```python
from build123d import *

# Parameters (mm, degrees)
ESQUISSE1_W        = 20
ESQUISSE1_H        = 7
BOSS_EXTRU_1_DEPTH = 23
ESQUISSE2_W        = 5
ESQUISSE2_H        = 2.5
BOSS_EXTRU_2_DEPTH = 2.5
ESQUISSE3_W        = 3
ESQUISSE3_H        = 3
ESQUISSE3_W_2      = 20
ESQUISSE3_H_2      = 7
BOSS_EXTRU_3_DEPTH = 2
CONG_1_R           = 2


with BuildPart() as part:
    # Esquisse1 → Boss.-Extru.1 (new body)
    with BuildSketch(Plane.XY):
        with Locations((10, 3.5)):
            Rectangle(ESQUISSE1_W, ESQUISSE1_H)
    extrude(amount=BOSS_EXTRU_1_DEPTH)

    # Esquisse2 → Boss.-Extru.2 (add)
    with BuildSketch(Plane.XY.offset(23)):
        with Locations((6.25, 3.5)):
            Rectangle(ESQUISSE2_W, ESQUISSE2_H)
        with Locations((13.75, 3.5)):
            Rectangle(ESQUISSE2_W, ESQUISSE2_H)
    extrude(amount=BOSS_EXTRU_2_DEPTH)

    # Esquisse3 → Boss.-Extru.3 (add)
    # profile 1 of 3: a face of its own
    with BuildSketch(Plane(origin=(0, 0, 0), x_dir=(-1, 0, 0), z_dir=(0, 0, -1))):
        with Locations((-21.5, 8.5)):
            Rectangle(ESQUISSE3_W, ESQUISSE3_H)
    # profile 2 of 3: a face of its own
    with BuildSketch(Plane(origin=(0, 0, 0), x_dir=(-1, 0, 0), z_dir=(0, 0, -1))):
        Polygon((-20, 10), (-20, 7), (-23, 7), (-23, -3), (3, -3), (3, 10), align=None)
        with Locations((-10, 3.5)):
            Rectangle(ESQUISSE3_W_2, ESQUISSE3_H_2, mode=Mode.SUBTRACT)
    # profile 3 of 3: a face of its own
    with BuildSketch(Plane(origin=(0, 0, 0), x_dir=(-1, 0, 0), z_dir=(0, 0, -1))):
        with Locations((-10, 3.5)):
            Rectangle(ESQUISSE3_W_2, ESQUISSE3_H_2)
    extrude(amount=BOSS_EXTRU_3_DEPTH)

    # Congé1
    cong_1_edges = [part.edges().sort_by_distance(p)[0] for p in [
        (10, 7, 0),
        (20, 3.5, 0),
        (10, 0, 0),
        (0, 3.5, 0),
    ]]
    fillet(cong_1_edges, radius=CONG_1_R)


solid = part.part
```
The model under review builds one solid part; all positions refer to its coordinate system, in mm. A direction names the side the tool comes from. Round coordinates to 2 decimals unless told otherwise and drop trailing zeros. Loops run counter-clockwise (first coordinate to the right, second up) from the corner with the lowest first, then second, coordinate; pieces in that order, holes last. Notation, with made-up numbers: (87.5, -22) - (142.5, -22) arc R7 ccw to (142.5, -10) - close; hole circle Ø3 at (8.5, -36). An arc over 180 degrees is marked (long way). Write each question's results on one line, items separated by ' | '. Start each with the question number.
Q1. Take a section at A-A on y = 2.75. Give the boundary of the cut face in (x, z).
Q2. Tool access review of faces 4 (the flat face through (6, 2.25, 24)), 5 (the flat face through (11, -2.2, 0)), 6 (the flat face through (3.75, 3, 24)): name each direction out of +Z, -Z, +X, -X, +Y, -Y from which nothing blocks a thin tool from reaching the whole face with its end or side.
Q3. Take a section at B-B on z = 23.75. Give the boundary of the cut face in (x, y).
Q4. Insertion check: P1, Ø3.5, axis at y = 4, z = 9.5, coming from the -X side; P2, Ø0.8, axis at x = 6, z = 24.5, coming from the -Y side; P3, Ø2, axis at x = 4.5, y = -1.5, coming from the +Z side. Each pin has a flat end and moves straight along its axis. Give the tip position at first contact, or say it passes through.
Q5. Take a section at D-D on y = 5.5. Give the boundary of the cut face in (x, z).
Q6. Wall thickness on line 1 along Y through (x, z) = (7, 17.5); line 2 along X through (y, z) = (1.5, 7); line 3 along Z through (x, y) = (3, 0.25): over which ranges is each line inside the solid? List them lowest first. Write a range as [from, to].
Q7. Take a section at C-C on x = 2. Give the boundary of the cut face in (y, z).
Q8. Draft analysis for pull direction X (two halves, no side actions). For faces 1 (the cylindrical face through (20.87, 3.58, 0.35)), 2 (the flat face through (10, 7, 12)), 3 (the flat face through (8.75, 3, 24)), state which applies: pulls with the +X half, pulls with the -X half, needs draft (parallel to the pull), parting line crosses it, or undercut.
Data:
1) outline: (-3, -2) - (23, -2) - (23, 0) - (22, 0) arc R2 cw to (20, 2) - (20, 23) - (16.25, 23) - (16.25, 25.5) - (11.25, 25.5) - (11.25, 23) - (8.75, 23) - (8.75, 25.5) - (3.75, 25.5) - (3.75, 23) - (0, 23) - (0, 2) arc R2 cw to (-2, 0) - (-3, 0) - close
2) face 4: +Z, +X, -X, -Y | face 5: +Z | face 6: +Z, -X, +Y, -Y
3) outline: (3.75, 2.25) - (8.75, 2.25) - (8.75, 4.75) - (3.75, 4.75) - close; (11.25, 2.25) - (16.25, 2.25) - (16.25, 4.75) - (11.25, 4.75) - close
4) P1: stops at x = 0 | P2: stops at y = 2.25 | P3: stops at z = 0.68
5) outline: (-3, -2) - (23, -2) - (23, 0) - (22, 0) arc R2 cw to (20, 2) - (20, 23) - (0, 23) - (0, 2) arc R2 cw to (-2, 0) - (-3, 0) - close
6) line 1: y = [0, 7] | line 2: x = [0, 20] | line 3: z = [-2, 23]
7) outline: (-3, -2) - (10, -2) - (10, 0) - (9, 0) arc R2 cw to (7, 2) - (7, 23) - (0, 23) - (0, 2) arc R2 cw to (-2, 0) - (-3, 0) - close
8) face 1: pulls with the +X half | face 2: needs draft | face 3: undercut
